Part print with two shaded views. Sizes in mm from the minimum x, y, z corner. A direction names the side the tool comes from. Round coordinates to 2 decimals unless told otherwise and drop trailing zeros. Loops run counter-clockwise (first coordinate to the right, second up) from the corner with the lowest first, then second, coordinate; pieces in that order, holes last. Notation, with made-up numbers: (-23, 22) - (-11, 22) arc R5 ccw to (-11, 27) - close; hole circle Ø6 at (-24.75, -6). An arc over 180 degrees is marked (long way). Use a Markdown table: item, result.
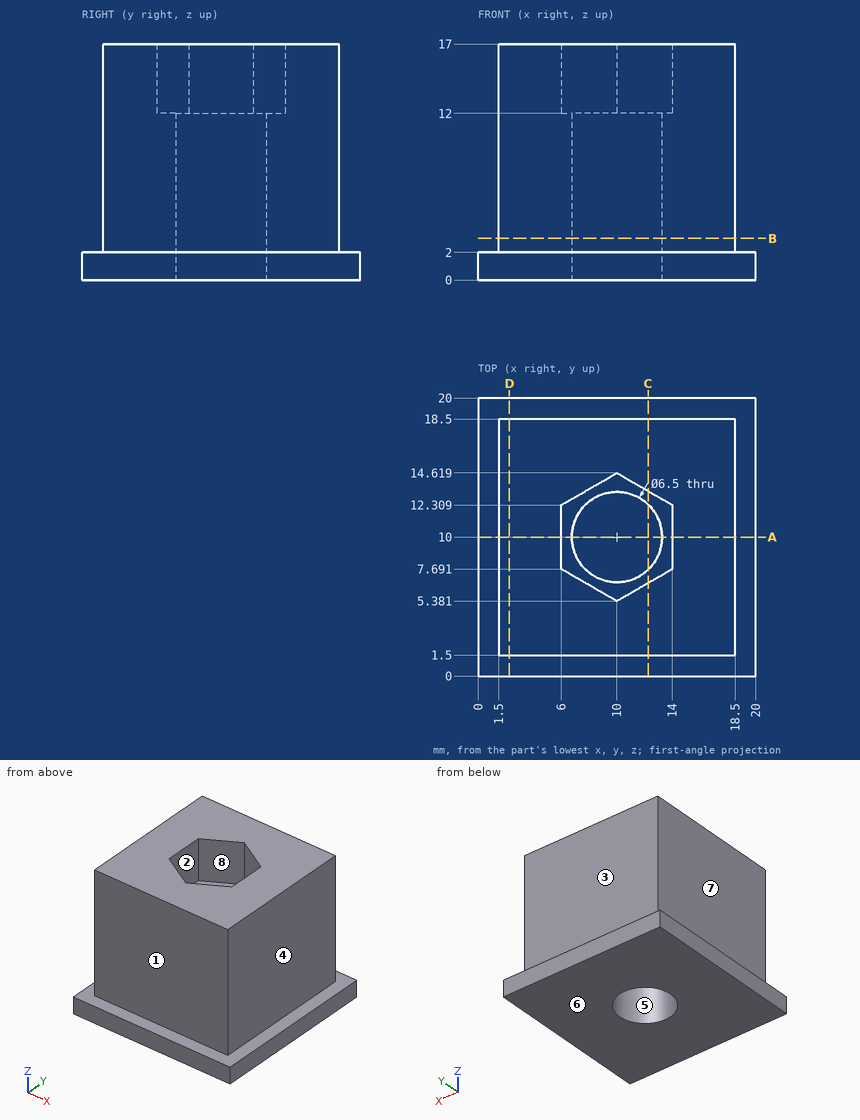
Q1. Pull direction X, two halves, no side cores. Call the marked faces 5, 6, 7 and 8: pulls with the +X half, pulls with the -X half, needs draft (parallel to the pull), parting line crosses it, or undercut.
Results found:
| item | result |
|---|---|
| face 5 | undercut |
| face 6 | needs draft |
| face 7 | pulls with the -X half |
| face 8 | undercut |
Q2. Cut at C-C, the plane x = 12.25. List the corners of the cut face in (y, z) (1 decimal).
Results found:
| item | result |
|---|---|
| outline | (0, 0) - (7.7, 0) - (7.7, 12) - (6.7, 12) - (6.7, 17) - (1.5, 17) - (1.5, 2) - (0, 2) - close; (12.3, 0) - (20, 0) - (20, 2) - (18.5, 2) - (18.5, 17) - (13.3, 17) - (13.3, 12) - (12.3, 12) - close |
Q3. Cut at B-B, the plane z = 3. List the corners of the cut face in (x, y), plus the area to 3 significant figures.
Results found:
| item | result |
|---|---|
| outline | (1.5, 1.5) - (18.5, 1.5) - (18.5, 18.5) - (1.5, 18.5) - close; hole circle Ø6.5 at (10, 10) |
| area | 256 mm2 |
Q4. Cut at D-D, the plane x = 2.25. List the corners of the cut face in (y, z), plus the area to 3 significant figures.
Results found:
| item | result |
|---|---|
| outline | (0, 0) - (20, 0) - (20, 2) - (18.5, 2) - (18.5, 17) - (1.5, 17) - (1.5, 2) - (0, 2) - close |
| area | 295 mm2 |
Q5. Probe line 1 (X direction, y = 10, z = 8.5); line 2 (Y direction, x = 14.25, z = 11.25). List the from-to ranges inside material, lowest first.
Results found:
| item | result |
|---|---|
| line 1 | x = 1.5 to 6.75, 13.25 to 18.5 |
| line 2 | y = 1.5 to 18.5 |
Q6. Cut at A-A, the plane y = 10. List the corners of the cut face in (x, z), plus the area to 3 significant figures.
Results found:
| item | result |
|---|---|
| outline | (0, 0) - (6.75, 0) - (6.75, 12) - (6, 12) - (6, 17) - (1.5, 17) - (1.5, 2) - (0, 2) - close; (13.25, 0) - (20, 0) - (20, 2) - (18.5, 2) - (18.5, 17) - (14, 17) - (14, 12) - (13.25, 12) - close |
| area | 177 mm2 |
Q7. Which spindle directions (+Z, -Z, +X, -X, +Y, -Y) get a long thin tool onto all of the face, cutting with end or side? Do the marked faces 1, 2, 3 and 4. Say none if no direction does.
Results found:
| item | result |
|---|---|
| face 1 | +Z, +X, -X, -Y |
| face 2 | +Z |
| face 3 | +Z, +X, -X, +Y |
| face 4 | +Z, +X, +Y, -Y |
Q8. Drop flat-ended pins along their axis: pin 1 (2 mm diameter, centred on y = 16, z = 7.5, fed in from +X); pin 2 (8 mm diameter, centred on x = 12.5, y = 12.5, fed in from -Z); pin 3 (2 mm diameter, centred on x = 11.5, z = 7.5, fed in from +Y); pin 4 (7.5 mm diameter, centred on y = 7, z = 6.5, fed in from -X). Give the stop position or say it passes through.
Results found:
| item | result |
|---|---|
| pin 1 | stops at x = 18.5 |
| pin 2 | stops at z = 0 |
| pin 3 | stops at y = 18.5 |
| pin 4 | stops at x = 1.5 |
